Could you check a few things on this drawing? It's one solid part, dimensions in mm from its lowest x, y, z. A direction names the side the tool comes from. Give positions to 0.01 mm unless a question says otherwise; leave off trailing zeros. Loops run counter-clockwise (first coordinate to the right, second up) from the corner with the lowest first, then second, coordinate; pieces in that order, holes last.
1. I need wall thicknesses on line 1 along X through (y, z) = (30, 25); line 2 along X through (y, z) = (9.5, 46.5); line 3 along Z through (x, y) = (20.5, 31.5). Which ranges of each line are inside material? Lowest first, please.
2. Imagine slicing it at C-C (y = 21.5). List the corners of the cut face in (x, z) for me.
3. Imagine slicing it at A-A (y = 13.5). List the corners of the cut face in (x, z) for me, plus the area to 3 significant figures.
4. Imagine slicing it at D-D (z = 16). List the corners of the cut face in (x, y) for me.
5. Thinking about a two-plate mould opening in X: for the marked faces 3, 4, 5 and 6, which applies, +X half, -X half, draft (parallel to the pull), parting line (faces both ways), or undercut?
6. For P1, Ø4, axis at x = 25, z = 42, coming from the -Y side; P2, Ø12, axis at x = 44, y = 58, coming from the -Z side; P3, Ø2, axis at x = 58.5, y = 59, coming from the -Z side (1 decimal), each with a flat end and sliding along its axis, tell me the tip position at first contact or that it passes through.
7. For the marked faces 1 and 2, which set-ups out of +Z, -Z, +X, -X, +Y, -Y let a thin tool reach every point of the face, with its end or its side?
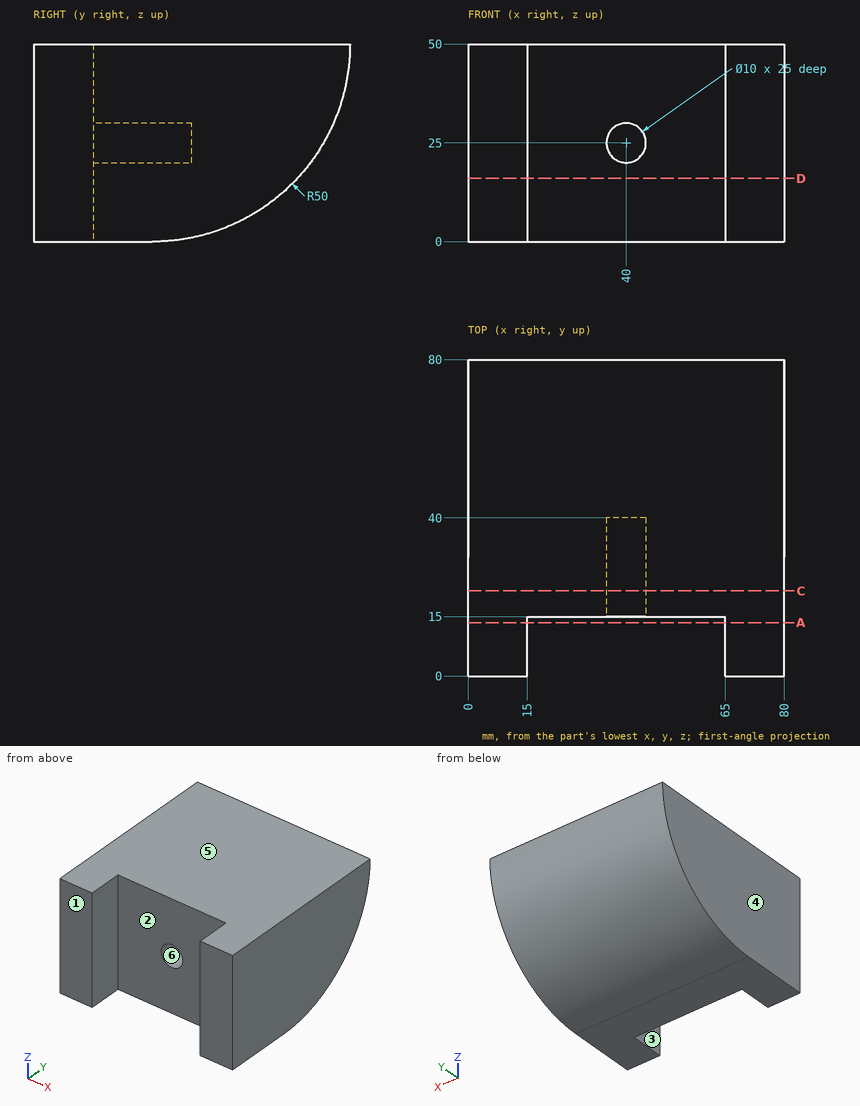
Derived:
1. line 1: x = 0 to 35, 45 to 80
1. line 2: x = 0 to 15, 65 to 80
1. line 3: z = 0.02 to 50
2. outline: (0, 0) - (80, 0) - (80, 50) - (0, 50) - close; hole circle Ø10 at (40, 25)
3. outline: (0, 0) - (15, 0) - (15, 50) - (0, 50) - close; (65, 0) - (80, 0) - (80, 50) - (65, 50) - close
3. area: 1,500 mm2
4. outline: (0, 0) - (15, 0) - (15, 15) - (65, 15) - (65, 0) - (80, 0) - (80, 66.66) - (0, 66.66) - close
5. face 3: undercut
5. face 4: -X half
5. face 5: draft
5. face 6: undercut
6. P1: stops at y = 15
6. P2: stops at z = 5.1
6. P3: stops at z = 8.6
7. face 1: +Z, -Z, +X, -X, -Y
7. face 2: +Z, -Z, -Y
